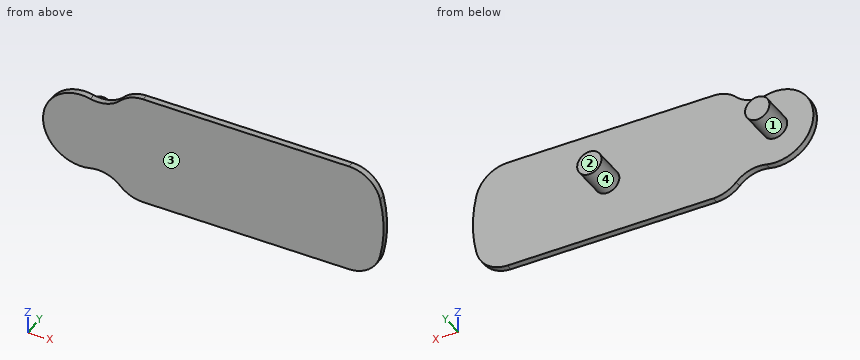
```python
from build123d import *

# Parameters (mm, degrees)
SKETCH1_R           = 12
SKETCH1_R_2         = 42
BOSS_EXTRUDE1_DEPTH = 2
SKETCH2_R           = 3.8
BOSS_EXTRUDE2_DEPTH = 10
FILLET1_R           = 10
CUT_EXTRUDE1_START  = -10
CUT_EXTRUDE1_DEPTH  = 10
FILLET2_R           = 10


with BuildPart() as part:
    # Sketch1 → Boss-Extrude1 (new body)
    with BuildSketch(Plane(origin=(0, 0, 0), x_dir=(1, 0, 0), z_dir=(0, 1, 0))):
        Circle(SKETCH1_R)
        with Locations((52.5, 0)):
            Circle(SKETCH1_R_2)
    extrude(amount=BOSS_EXTRUDE1_DEPTH)

    # Sketch2 → Boss-Extrude2 (add)
    with BuildSketch(Plane(origin=(0, 2, 0), x_dir=(1, 0, 0), z_dir=(0, 1, 0))):
        with Locations(Location((0, 0, 0), (0, 0, 270))):
            Circle(SKETCH2_R)
        with Locations(Location((52.5, 0, 0), (0, 0, 270))):
            Circle(SKETCH2_R)
    extrude(amount=BOSS_EXTRUDE2_DEPTH)

    # Fillet1
    fillet1_edges = [part.edges().sort_by_distance(p)[0] for p in [
        (10.821428571, 1, 5.186201276),
        (10.821428571, 1, -5.186201276),
    ]]
    fillet(fillet1_edges, radius=FILLET1_R)

    # Sketch3 → Cut-Extrude1 (cut)
    with BuildSketch(Plane(origin=(0, 2, 0), x_dir=(1, 0, 0), z_dir=(0, 1, 0)).offset(CUT_EXTRUDE1_START)):
        with BuildLine():
            Line((14.221153846, -17.283805632), (90.778846154, -17.283805632))
            ThreePointArc((90.778846154, -17.283805632), (52.5, -42), (14.221153846, -17.283805632))
        make_face()
        with BuildLine():
            Line((14.221153846, 17.283805632), (90.778846154, 17.283805632))
            ThreePointArc((90.778846154, 17.283805632), (52.5, 42), (14.221153846, 17.283805632))
        make_face()
    extrude(amount=CUT_EXTRUDE1_DEPTH, mode=Mode.SUBTRACT)

    # Fillet2
    fillet2_edges = [part.edges().sort_by_distance(p)[0] for p in [
        (14.221153846, 1, 17.283805632),
        (14.221153846, 1, -17.283805632),
        (90.778846154, 1, 17.283805632),
        (90.778846154, 1, -17.283805632),
    ]]
    fillet(fillet2_edges, radius=FILLET2_R)


solid = part.part
```
Source: CAD feature listing. Evaluate the final solid. Frame: model axes, mm. Face numbers are marked on the shaded views. A direction names the side the tool comes from. Give positions to 0.01 mm unless a question says otherwise; leave off trailing zeros. Write each loop counter-clockwise with the first axis right and the second up, starting at its lowest first coordinate (ties: lowest second). Pieces come first, ordered by that corner, then holes.
1. First-contact query: pin 1 (3 mm diameter, centred on x = 76.5, z = -1.5, fed in from +Y). Flat tip, straight axial feed; report the tip coordinate or a pass-through.
2. Material intervals for line 1 along Y through (x, z) = (46, 6); line 2 along X through (y, z) = (9, 1); line 3 along X through (y, z) = (6.5, 0.5), sorted ascending.
3. Section query B-B (y = 10.5). Return the cut outline in (x, z).
4. Pull-direction query (X, two-part tool) for the marked faces 1 and 2; classes: +X half, -X half, draft (parallel to the pull), parting line (faces both ways), or undercut.
5. Access query for the marked faces 3 and 4. Directions: +Z, -Z, +X, -X, +Y, -Y. A direction counts if a zero-diameter tool reaches every point of the face in a straight line with its end or side. Return the directions, or none.
6. Section query D-D (x = 52.5). Return the cut outline in (y, z), then the cut area to 3 significant figures.
7. Section query A-A (x = 0). Return the cut outline in (y, z), then the cut area to 3 significant figures.
8. Section query C-C (z = 0). Return the cut outline in (x, y), then the cut area to 3 significant figures.
Output values:
1. pin 1: stops at y = 2
2. line 1: y = 0 to 2
2. line 2: x = -3.67 to 3.67, 48.83 to 56.17
2. line 3: x = -3.77 to 3.77, 48.73 to 56.27
3. outline: circle Ø7.6 at (0, 0); circle Ø7.6 at (52.5, 0)
4. face 1: undercut
4. face 2: draft
5. face 3: +Z, -Z, +X, -X, -Y
5. face 4: +Y
6. outline: (0, -17.28) - (2, -17.28) - (2, -3.8) - (12, -3.8) - (12, 3.8) - (2, 3.8) - (2, 17.28) - (0, 17.28) - close
6. area: 145 mm2
7. outline: (0, -12) - (2, -12) - (2, -3.8) - (12, -3.8) - (12, 3.8) - (2, 3.8) - (2, 12) - (0, 12) - close
7. area: 124 mm2
8. outline: (-12, 0) - (94.5, 0) - (94.5, 2) - (56.3, 2) - (56.3, 12) - (48.7, 12) - (48.7, 2) - (3.8, 2) - (3.8, 12) - (-3.8, 12) - (-3.8, 2) - (-12, 2) - close
8. area: 365 mm2
